Source: three-view drawing plus pictorial views. Frame: mm from the lowest corner of the part. Coordinates: 2 decimals unless noted, no trailing zeros. Write each loop counter-clockwise with the first axis right and the second up, starting at its lowest first coordinate (ties: lowest second). Pieces come first, ordered by that corner, then holes. Notation, with made-up numbers: M 82,25 L 93,25 A10 cw 93,40 Z; hole C -25.5,-34 d1. An arc over 180 degrees is marked long. Write item = value, one per line. Start each with the question number.
Item 1: Section B-B on x = 27. Output: boundary loops of the cut face in (y, z) (1 decimal), plus the area to 3 significant figures.
Item 2: Ray query, L1, parallel to X at y = 69.5, z = 1.75 (1 decimal); L2, parallel to Y at x = 33, z = 1.9 (1 decimal); L3, parallel to Y at x = 25, z = 2.1 (1 decimal). Return the intervals inside material, ascending. Write a range as [from, to].
Item 3: First-contact query: pin 1 Ø6 at (x, y) = (16.5, 14) entering from -Z. Flat tip, straight axial feed; report the tip coordinate or a pass-through.
Item 4: Section A-A on y = 42. Output: boundary loops of the cut face in (x, z) (1 decimal).
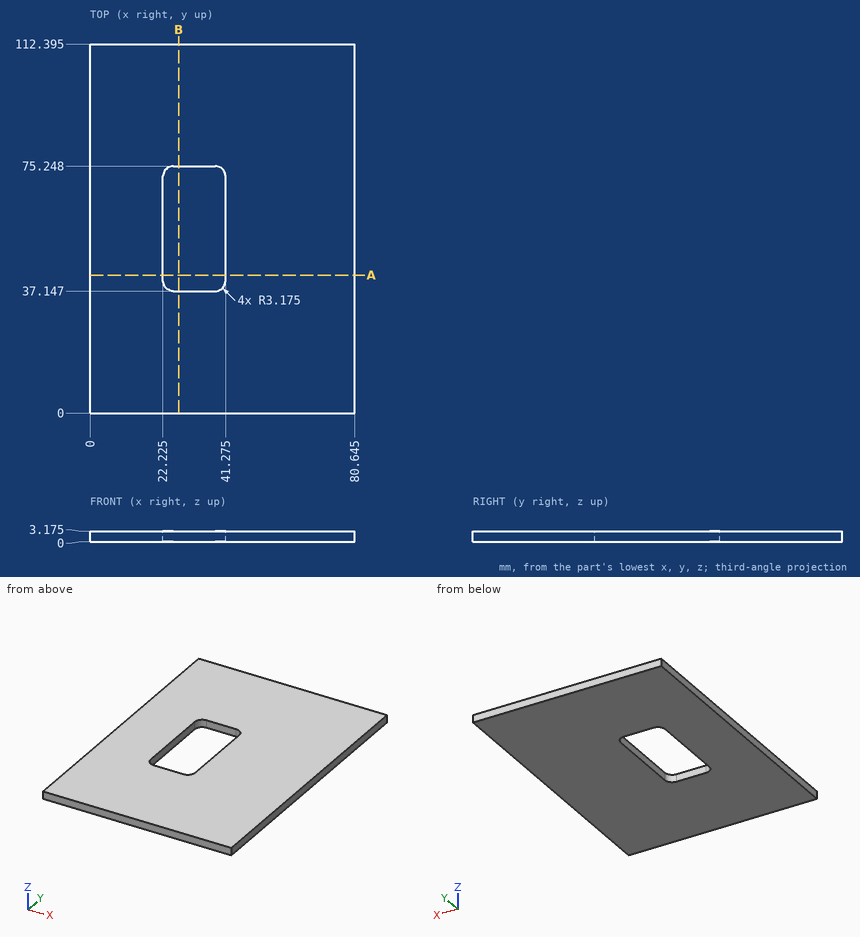
Responses:
q1.outline = M 0,0 L 37.1,0 L 37.1,3.2 L 0,3.2 Z; M 75.2,0 L 112.4,0 L 112.4,3.2 L 75.2,3.2 Z
q1.area = 236 mm²
q2.L1 = [0, 22.2], [41.3, 80.6]
q2.L2 = [0, 37.1], [75.2, 112.4]
q2.L3 = [0, 37.2], [75.2, 112.4]
q3.pin_1 = 0
q4.outline = M 0,0 L 22.2,0 L 22.2,3.2 L 0,3.2 Z; M 41.3,0 L 80.6,0 L 80.6,3.2 L 41.3,3.2 Z
